from build123d import *

# Parameters (mm, degrees)
F0_W     = 215.9
F0_H     = 215.9
F1_DEPTH = 2.54
F3_DEPTH = 12.7
F6_COUNT = 4
F6_ANGLE = 270
F7_DEPTH = 25.401


with BuildPart() as f1:
    # F0 (on Top) → F1 (new body)
    with BuildSketch(Plane.XY):
        Rectangle(F0_W, F0_H)
    extrude(amount=-F1_DEPTH)


with BuildPart() as f3:
    # F2 (on face) → F3 (new body, symmetric)
    with BuildSketch(Plane.XY):
        Polygon((-76.2, -107.95), (0, -107.95), (0, -95.25), (-63.4950530427, -94.4573846459), align=None)
    extrude(amount=F3_DEPTH, both=True)


with BuildPart() as f4_1:
    # F4: instance of F3
    add(f3.part.mirror(Plane.YZ))


with BuildPart() as f6_1:
    # F6: instance of F3
    add(f3.part.rotate(Axis((0, 0, 47.5433133543), (0, 0, 1)), 1 * F6_ANGLE / (F6_COUNT - 1)))


with BuildPart() as f6_2:
    # F6: instance of F3
    add(f3.part.rotate(Axis((0, 0, 47.5433133543), (0, 0, 1)), 2 * F6_ANGLE / (F6_COUNT - 1)))


with BuildPart() as f6_3:
    # F6: instance of F3
    add(f3.part.rotate(Axis((0, 0, 47.5433133543), (0, 0, 1)), 3 * F6_ANGLE / (F6_COUNT - 1)))


with BuildPart() as f6_4:
    # F6: instance of F4_1
    add(f4_1.part.rotate(Axis((0, 0, 47.5433133543), (0, 0, 1)), 1 * F6_ANGLE / (F6_COUNT - 1)))


with BuildPart() as f6_5:
    # F6: instance of F4_1
    add(f4_1.part.rotate(Axis((0, 0, 47.5433133543), (0, 0, 1)), 2 * F6_ANGLE / (F6_COUNT - 1)))


with BuildPart() as f6_6:
    # F6: instance of F4_1
    add(f4_1.part.rotate(Axis((0, 0, 47.5433133543), (0, 0, 1)), 3 * F6_ANGLE / (F6_COUNT - 1)))


with BuildPart() as f7_tool:
    # F6_face (on face) + F4_face (on face) + F3_face (on face) → F7 (new body, through all)
    with BuildSketch(Plane(origin=(-35.4001438313, 101.5916492403, 12.7), x_dir=(1, 0, 0), z_dir=(0, 0, 1))):
        Polygon((-40.7998561687, 6.3583507597), (-28.0949092115, -7.1342645945), (35.4001438313, -6.3416492403), (35.4001438313, 6.3583507597), align=None)
        Polygon((98.895196874, -7.1342645945), (111.6001438313, 6.3583507597), (35.4001438313, 6.3583507597), (35.4001438313, -6.3416492403), align=None)
        Polygon((143.3501438313, -25.3916492403), (129.8575284771, -38.0965961976), (130.6501438313, -101.5916492403), (143.3501438313, -101.5916492403), align=None)
        Polygon((129.8575284771, -165.0867022831), (143.3501438313, -177.7916492403), (143.3501438313, -101.5916492403), (130.6501438313, -101.5916492403), align=None)
        Polygon((-72.5498561687, -177.7916492403), (-59.0572408146, -165.0867022831), (-59.8498561687, -101.5916492403), (-72.5498561687, -101.5916492403), align=None)
        Polygon((-59.0572408146, -38.0965961976), (-72.5498561687, -25.3916492403), (-72.5498561687, -101.5916492403), (-59.8498561687, -101.5916492403), align=None)
    with BuildSketch(Plane(origin=(35.4001438313, -101.5916492403, 12.7), x_dir=(1, 0, 0), z_dir=(0, 0, 1))):
        Polygon((40.7998561687, -6.3583507597), (28.0949092115, 7.1342645945), (-35.4001438313, 6.3416492403), (-35.4001438313, -6.3583507597), align=None)
    with BuildSketch(Plane(origin=(-35.4001438313, -101.5916492403, 12.7), x_dir=(1, 0, 0), z_dir=(0, 0, 1))):
        Polygon((-28.0949092115, 7.1342645945), (-40.7998561687, -6.3583507597), (35.4001438313, -6.3583507597), (35.4001438313, 6.3416492403), align=None)
    extrude(amount=-F7_DEPTH)


with BuildPart() as f1_1:
    add(f1.part)

    # F7: cut by f7_tool
    add(f7_tool.part, mode=Mode.SUBTRACT)


with BuildPart() as f3_1:
    add(f3.part)

    # F7: cut by f7_tool
    add(f7_tool.part, mode=Mode.SUBTRACT)


with BuildPart() as f4_1_1:
    add(f4_1.part)

    # F7: cut by f7_tool
    add(f7_tool.part, mode=Mode.SUBTRACT)


with BuildPart() as f6_1_1:
    add(f6_1.part)

    # F7: cut by f7_tool
    add(f7_tool.part, mode=Mode.SUBTRACT)


with BuildPart() as f6_2_1:
    add(f6_2.part)

    # F7: cut by f7_tool
    add(f7_tool.part, mode=Mode.SUBTRACT)


with BuildPart() as f6_3_1:
    add(f6_3.part)

    # F7: cut by f7_tool
    add(f7_tool.part, mode=Mode.SUBTRACT)


with BuildPart() as f6_4_1:
    add(f6_4.part)

    # F7: cut by f7_tool
    add(f7_tool.part, mode=Mode.SUBTRACT)


with BuildPart() as f6_5_1:
    add(f6_5.part)

    # F7: cut by f7_tool
    add(f7_tool.part, mode=Mode.SUBTRACT)


with BuildPart() as f6_6_1:
    add(f6_6.part)

    # F7: cut by f7_tool
    add(f7_tool.part, mode=Mode.SUBTRACT)


solid = f1_1.part
CAD build for the part. Positions are in the model's coordinates, mm. A direction names the side the tool comes from. Give positions to 0.01 mm unless a question says otherwise; leave off trailing zeros. Order: outer loops, then holes, each group sorted by start corner. A loop starts at its lowest first (then second) coordinate and runs counter-clockwise, first axis right, second up. Notation, with made-up numbers: (-24.5, -22) - (8.5, -22) arc R16 cw to (8.5, -6) - close; hole circle Ø6 at (-27, 1). An arc over 180 degrees is marked (long way). Answer in a Markdown table with one row per item.
1. Saw through at C-C, the plane x = -23. Give the cut face in (y, z).
Data:
| item | result |
|---|---|
| outline | (-94.96, -2.54) - (94.96, -2.54) - (94.96, 0) - (-94.96, 0) - close |
2. Pull direction X, two halves, no side cores. Call faces 4 (the flat face through (-101.11, 69.76, -1.25)), 5 (the flat face through (-69.94, 101.3, -1.25)), 6 (the flat face through (101.11, -69.76, -1.25)), 7 (the flat face through (69.94, -101.3, -1.25)): pulls with the +X half, pulls with the -X half, needs draft (parallel to the pull), parting line crosses it, or undercut.
Data:
| item | result |
|---|---|
| face 4 | pulls with the -X half |
| face 5 | undercut |
| face 6 | pulls with the +X half |
| face 7 | undercut |
3. Saw through at B-B, the plane y = 68. Give the cut face in (x, z), plus the area to 3 significant figures.
Data:
| item | result |
|---|---|
| outline | (-99.24, -2.54) - (99.24, -2.54) - (99.24, 0) - (-99.24, 0) - close |
| area | 504 mm² |
4. Saw through at A-A, the plane z = -1.6. Give the cut face in (x, y).
Data:
| item | result |
|---|---|
| outline | (-107.95, -107.95) - (-76.2, -107.95) - (-63.5, -94.46) - (0, -95.25) - (63.5, -94.46) - (76.2, -107.95) - (107.95, -107.95) - (107.95, -76.2) - (94.46, -63.5) - (95.25, 0) - (94.46, 63.5) - (107.95, 76.2) - (107.95, 107.95) - (76.2, 107.95) - (63.5, 94.46) - (0, 95.25) - (-63.5, 94.46) - (-76.2, 107.95) - (-107.95, 107.95) - (-107.95, 76.2) - (-94.46, 63.5) - (-95.25, 0) - (-94.46, -63.5) - (-107.95, -76.2) - close |
5. Tool access for faces 1 (the flat face through (-101.3, -69.94, -1.25)), 2 (the flat face through (101.3, 69.94, -1.25)), 3 (the flat face through (69.76, 101.11, -1.25)): list every direction of +Z, -Z, +X, -X, +Y, -Y with a clear straight run to the whole face (end or side of a thin tool).
Data:
| item | result |
|---|---|
| face 1 | +Z, -Z, -X |
| face 2 | +Z, -Z, +X |
| face 3 | +Z, -Z, +Y |
6. Flat gauge pin, fed straight in: pin 1 (1 mm diameter, centred on x = 51, z = -0.5, fed in from +Y). Where does the tip first touch, or does it go through?
Data:
| item | result |
|---|---|
| pin 1 | stops at y = 94.62 |
7. Probe probe 1 along Y at (x, z) = (60.5, -2.1); probe 2 along X at (y, z) = (2, -2.25); probe 3 along Y at (x, z) = (-2.5, -1.9). List the from-to ranges inside material, lowest first. Write a range as [from, to].
Data:
| item | result |
|---|---|
| probe 1 | y = [-94.49, 94.49] |
| probe 2 | x = [-95.23, 95.23] |
| probe 3 | y = [-95.22, 95.22] |
